Build history of the part. All positions in model axes, mm. Round coordinates to 2 decimals unless told otherwise and drop trailing zeros. Write each loop counter-clockwise with the first axis right and the second up, starting at its lowest first coordinate (ties: lowest second). Pieces come first, ordered by that corner, then holes. Notation, with made-up numbers: (19, -33.5) -> (34, -33.5) arc R18 cw to (34, -25.5) -> close; hole circle Ø8 at (-11, 45). An arc over 180 degrees is marked (long way). Answer in a Markdown table with one row per item.
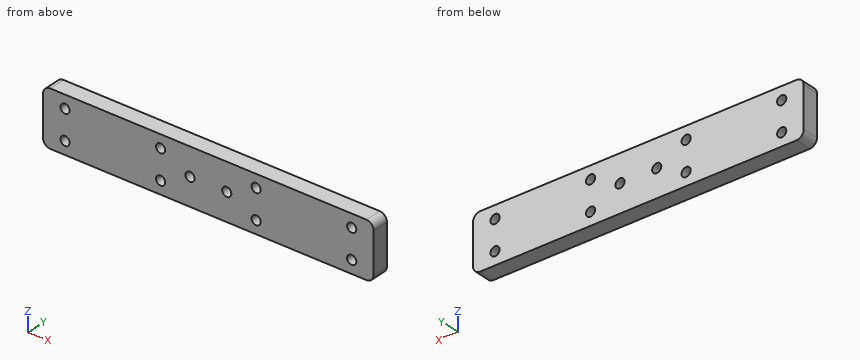
```python
from build123d import *

# Parameters (mm, degrees)
SKETCH_1_R      = 1.25
EXTRUDE_1_DEPTH = 4.5


with BuildPart() as part:
    # 草图1 → 凸台-拉伸1 (new body)
    with BuildSketch(Plane(origin=(0, 0, 0), x_dir=(1, 0, 0), z_dir=(0, 1, 0))):
        with BuildLine():
            Line((-43, 7.5), (43, 7.5))
            ThreePointArc((43, 7.5), (44.414213562, 6.914213562), (45, 5.5))
            Line((45, 5.5), (45, -5.5))
            ThreePointArc((45, -5.5), (44.414213562, -6.914213562), (43, -7.5))
            Line((43, -7.5), (-43, -7.5))
            ThreePointArc((-43, -7.5), (-44.414213562, -6.914213562), (-45, -5.5))
            Line((-45, -5.5), (-45, 5.5))
            ThreePointArc((-45, 5.5), (-44.414213562, 6.914213562), (-43, 7.5))
        make_face()
        with Locations(Location((-5, 0, 0), (0, 0, 270))):
            Circle(SKETCH_1_R, mode=Mode.SUBTRACT)
        with Locations(Location((5, 0, 0), (0, 0, 270))):
            Circle(SKETCH_1_R, mode=Mode.SUBTRACT)
        with Locations(Location((-39, 4, 0), (0, 0, 270))):
            Circle(SKETCH_1_R, mode=Mode.SUBTRACT)
        with Locations(Location((-39, -4, 0), (0, 0, 270))):
            Circle(SKETCH_1_R, mode=Mode.SUBTRACT)
        with Locations(Location((-13, -4, 0), (0, 0, 270))):
            Circle(SKETCH_1_R, mode=Mode.SUBTRACT)
        with Locations(Location((-13, 4, 0), (0, 0, 270))):
            Circle(SKETCH_1_R, mode=Mode.SUBTRACT)
        with Locations(Location((13, -4, 0), (0, 0, 270))):
            Circle(SKETCH_1_R, mode=Mode.SUBTRACT)
        with Locations(Location((13, 4, 0), (0, 0, 270))):
            Circle(SKETCH_1_R, mode=Mode.SUBTRACT)
        with Locations(Location((39, -4, 0), (0, 0, 270))):
            Circle(SKETCH_1_R, mode=Mode.SUBTRACT)
        with Locations(Location((39, 4, 0), (0, 0, 270))):
            Circle(SKETCH_1_R, mode=Mode.SUBTRACT)
    extrude(amount=EXTRUDE_1_DEPTH)


solid = part.part
```
Q1. Saw through at B-B on y = 3.3. State how many separate pieces and enclosed holes the cut face has, plus the area to 3 significant figures.
A:
| item | result |
|---|---|
| separate pieces | 1 |
| enclosed holes | 10 |
| area | 1,300 mm² |
Q2. Drop a flat-ended pin along its axis: P1, Ø2, axis at x = -13, z = 4, coming from the +Y side. Give the stop position or say it passes through.
A:
| item | result |
|---|---|
| P1 | through |
Q3. Saw through at C-C on z = 4. Write the cut outline in (x, y).
A:
| item | result |
|---|---|
| outline | (-45, 0) -> (-40.25, 0) -> (-40.25, 4.5) -> (-45, 4.5) -> close; (-37.75, 0) -> (-14.25, 0) -> (-14.25, 4.5) -> (-37.75, 4.5) -> close; (-11.75, 0) -> (11.75, 0) -> (11.75, 4.5) -> (-11.75, 4.5) -> close; (14.25, 0) -> (37.75, 0) -> (37.75, 4.5) -> (14.25, 4.5) -> close; (40.25, 0) -> (45, 0) -> (45, 4.5) -> (40.25, 4.5) -> close |
Q4. Saw through at D-D on z = 0. Write the cut outline in (x, y).
A:
| item | result |
|---|---|
| outline | (-45, 0) -> (-6.25, 0) -> (-6.25, 4.5) -> (-45, 4.5) -> close; (-3.75, 0) -> (3.75, 0) -> (3.75, 4.5) -> (-3.75, 4.5) -> close; (6.25, 0) -> (45, 0) -> (45, 4.5) -> (6.25, 4.5) -> close |
Q5. Wall check: line 1 (X direction, y = 2, z = 0); line 2 (X direction, y = 1.95, z = 4); line 3 (X direction, y = 1.25, z = 3.25). Give the ranges that are in metal, low to high. Write a range as [from, to].
A:
| item | result |
|---|---|
| line 1 | [-45, -6.25], [-3.75, 3.75], [6.25, 45] |
| line 2 | [-45, -40.25], [-37.75, -14.25], [-11.75, 11.75], [14.25, 37.75], [40.25, 45] |
| line 3 | [-45, -40], [-38, -14], [-12, 12], [14, 38], [40, 45] |
Q6. Saw through at A-A on x = 13. Write the cut outline in (y, z), plus the area to 3 significant figures.
A:
| item | result |
|---|---|
| outline | (0, -7.5) -> (4.5, -7.5) -> (4.5, -5.25) -> (0, -5.25) -> close; (0, -2.75) -> (4.5, -2.75) -> (4.5, 2.75) -> (0, 2.75) -> close; (0, 5.25) -> (4.5, 5.25) -> (4.5, 7.5) -> (0, 7.5) -> close |
| area | 45.0 mm² |
